```python
from build123d import *

# Parameters (mm, degrees)
F1_DEPTH = 127
F0_R     = 50.8
F2_DEPTH = 50.8
F3_DEPTH = 76.2


with BuildPart() as f1:
    # F0 (on Front) → F1 (new body)
    with BuildSketch(Plane.XZ):
        Polygon((8.923398, -12.435868), (69.251364, -12.435868), (69.251364, 49.901095), (-184.748636, 49.901095), (-184.748636, -13.598905), (-118.076602, -13.598905), (-156.176602, 24.501095), (45.860362, 24.501095), align=None)
    extrude(amount=F1_DEPTH)

    # F0 (on Front) → F2 (join)
    with BuildSketch(Plane.XZ):
        with BuildLine():
            Line((-184.748636, 49.901095), (69.251364, 49.901095))
            Line((69.251364, 49.901095), (25.984603, 171.206705))
            ThreePointArc((25.984603, 171.206705), (29.850151, 156.495716), (31.151364, 141.341095))
            ThreePointArc((31.151364, 141.341095), (-72.903256, 53.742308), (-141.481875, 171.206705))
            Line((-141.481875, 171.206705), (-184.748636, 49.901095))
        make_face()
        with BuildLine():
            ThreePointArc((31.151364, 141.341095), (29.850151, 156.495716), (25.984603, 171.206705))
            ThreePointArc((25.984603, 171.206705), (-57.748636, 230.241095), (-141.481875, 171.206705))
            ThreePointArc((-141.481875, 171.206705), (-72.903256, 53.742308), (31.151364, 141.341095))
        make_face()
        with Locations((-57.748636, 141.341095)):
            Circle(F0_R, mode=Mode.SUBTRACT)
    extrude(amount=F2_DEPTH)

    # F0 (on Front) → F3 (join)
    with BuildSketch(Plane.XZ):
        with BuildLine():
            ThreePointArc((31.151364, 141.341095), (29.850151, 156.495716), (25.984603, 171.206705))
            ThreePointArc((25.984603, 171.206705), (-57.748636, 230.241095), (-141.481875, 171.206705))
            ThreePointArc((-141.481875, 171.206705), (-72.903256, 53.742308), (31.151364, 141.341095))
        make_face()
        with Locations((-57.748636, 141.341095)):
            Circle(F0_R, mode=Mode.SUBTRACT)
    extrude(amount=F3_DEPTH)


solid = f1.part
```
The listing builds one solid part. Answer for the finished solid, in the listing's coordinates (mm). A direction names the side the tool comes from. Coordinates: 2 decimals unless noted, no trailing zeros. Write each loop counter-clockwise with the first axis right and the second up, starting at its lowest first coordinate (ties: lowest second). Pieces come first, ordered by that corner, then holes. Notation, with made-up numbers: M 64.5,-17.5 L 93.5,-17.5 A29 ccw 93.5,10.5 Z; hole C 83.5,28 d5. An arc over 180 degrees is marked long. Use a Markdown table: item, result. Add a question column.
1. Section C-C (z = 106.5) is taken. Give the vertices of the cut face in (x, y).
2. Straight lines are drawn through the part: line 1 along Z through (x, y) = (-101, -74.5); line 2 along Y through (x, z) = (-113, 182); line 3 along X through (y, z) = (-103, 21.5). For each, find the intervals that lie inside material, in ascending order. Write a range as [from, to].
3. Given P1, Ø4, axis at x = -93, y = -73, coming from the -Z side; P2, Ø4, axis at x = -10, y = -61, coming from the +Z side; P3, Ø10, axis at y = -53.5, z = 60, coming from the -X side, each flat-ended and moving along its own axis, determine where each tip first touches the part or whether it passes through.
4. Section A-A (y = -68.5) is taken. Give the vertices of the cut face in (x, z), plus the area to 3 significant figures.
5. Section D-D (y = -43) is taken. Give the vertices of the cut face in (x, z), plus the area to 3 significant figures.
6. Section B-B (x = -70) is taken. Give the vertices of the cut face in (y, z).
7. Which of the six approach directions +Z, -Z, +X, -X, +Y, -Y give full straight-line access (tool end or side, diameter ignored) to faces 4 (the flat face through (27.65, -62.61, 6.29)), 5 (the cylindrical face through (29.886, -63.322, 156.286)), 6 (the flat face through (-56, -88, 49.901))?
8. For a pull along Z with two mould halves and no side action, classify faces 1 (the flat face through (-162.812, -25.044, 111.403)), 2 (the flat face through (-49, -50.8, 52)), 3 (the flat face through (39, -63, -12.436)) as +Z half, -Z half, draft (parallel to the pull), parting line (faces both ways), or undercut.
Data:
| question | item | result |
|---|---|---|
| 1 | outline | M -164.56,-50.8 L -139.54,-50.8 L -139.54,-76.2 L -94.72,-76.2 L -94.72,0 L -164.56,0 Z; M -20.78,-76.2 L 24.04,-76.2 L 24.04,-50.8 L 49.06,-50.8 L 49.06,0 L -20.78,0 Z |
| 2 | line 1 | z = [24.5, 49.9], [63.67, 114.7], [167.99, 219.01] |
| 2 | line 2 | y = [-76.2, 0] |
| 2 | line 3 | x = [-184.75, -153.18], [42.86, 69.25] |
| 3 | P1 | stops at z = 24.5 |
| 3 | P2 | stops at z = 217.57 |
| 3 | P3 | stops at x = -182.65 |
| 4 | outline | M -184.75,-13.6 L -118.08,-13.6 L -156.18,24.5 L 45.86,24.5 L 8.92,-12.44 L 69.25,-12.44 L 69.25,49.9 L -184.75,49.9 Z; M 25.98,171.21 A88.9 ccw long 31.15,141.34 A88.9 ccw Z; hole C -57.75,141.34 d101.6 |
| 4 | area | 26,500 mm2 |
| 5 | outline | M -184.75,-13.6 L -118.08,-13.6 L -156.18,24.5 L 45.86,24.5 L 8.92,-12.44 L 69.25,-12.44 L 69.25,49.9 L 25.98,171.21 A88.9 ccw -141.48,171.21 L -184.75,49.9 Z; hole C -57.75,141.34 d101.6 |
| 5 | area | 34,500 mm2 |
| 6 | outline | M -127,24.5 L 0,24.5 L 0,92.04 L -76.2,92.04 L -76.2,53.29 L -50.8,53.29 L -50.8,49.9 L -127,49.9 Z; M -76.2,190.64 L 0,190.64 L 0,229.39 L -76.2,229.39 Z |
| 7 | face 4 | +Y, -Y |
| 7 | face 5 | +Z, +X, -Y |
| 7 | face 6 | +X, -X, -Y |
| 8 | face 1 | +Z half |
| 8 | face 2 | undercut |
| 8 | face 3 | -Z half |
